Geometry check sheet. Reference: the model listing, model coordinates, mm. Coordinates: 2 decimals unless noted, no trailing zeros. Write each loop counter-clockwise with the first axis right and the second up, starting at its lowest first coordinate (ties: lowest second). Pieces come first, ordered by that corner, then holes. Notation, with made-up numbers: M -0.5,0 L 18.5,0 A38 cw 18.5,38 Z; hole C 13,-30.5 d11. An arc over 180 degrees is marked long. Put each result on its own line as item: value. Start each with the question number.
1) Cross-section at B-B on x = 11. Record the cut outline in (y, z).
2) Cross-section at A-A on y = 2. Record the cut outline in (x, z).
3) Gauge pin test, flat end, axial feed: pin 1 (1.8 mm diameter, centred on x = -7.78, y = 7.78, fed in from +Z). Record the tip position at first contact, or that the pin passes through.
4) Cross-section at C-C on z = 0.4. Count the separate pieces of the cut face and the enclosed holes in it, plus the area to 3 significant figures.
5) Cross-section at D-D on x = 1. Record the cut outline in (y, z), plus the area to 3 significant figures.
6) Scan lines: line 1 along Y through (x, z) = (0, 0.2); line 2 along X through (y, z) = (7.5, 0.2); line 3 along X through (y, z) = (-1, 0.5). Record each from-to range of solid material in increasing order.
Autodesk Inventor part; units mm, degrees
ref_plane "YZ Plane" through (0, 0, 0) normal (1, 0, 0) x (0, 1, 0)
ref_plane "XZ Plane" through (0, 0, 0) normal (0, 1, 0) x (-1, 0, 0)
ref_plane "XY Plane" through (0, 0, 0) normal (0, 0, 1) x (1, 0, 0)
sketch "Sketch1" plane through (0, 0, 0) normal (0, 0, 1) x (1, 0, 0)
  line L0 (-13, -11) -> (13, -11) construction
  circle A0 centre (0, 0) radius 13.8 construction
  circle A1 centre (0, 0) radius 5 construction
  circle A2 centre (0, -11) radius 1.2813 construction
  circle A3 centre (-7.7782, -7.7782) radius 1.2813 construction
  circle A4 centre (-11, 0) radius 1.2813 construction
  circle A5 centre (-7.7782, 7.7782) radius 1.2813 construction
  circle A6 centre (0, 11) radius 1.2813 construction
  circle A7 centre (7.7782, 7.7782) radius 1.2813 construction
  circle A8 centre (11, 0) radius 1.2813 construction
  circle A9 centre (7.7782, -7.7782) radius 1.2813 construction
  circle A10 centre (0, -8) radius 1.2 construction
  circle A11 centre (-8, 0) radius 1.2 construction
  circle A12 centre (0, 8) radius 1.2 construction
  circle A13 centre (8, 0) radius 1.2 construction
  circle A14 centre (0, -11) radius 1.5
  circle A15 centre (7.7782, -7.7782) radius 1.5
  circle A16 centre (11, 0) radius 1.5
  circle A17 centre (7.7782, 7.7782) radius 1.5
  circle A18 centre (0, 11) radius 1.5
  circle A19 centre (-7.7782, 7.7782) radius 1.5
  circle A20 centre (-11, 0) radius 1.5
  circle A21 centre (-7.7782, -7.7782) radius 1.5
  circle A22 centre (0, 0) radius 6
  circle A23 centre (0, 0) radius 19
  dimension "d0" = 3
  dimension "d3" = 360
  dimension "d5" = 12
  dimension "d6" = 38
extrude "Extrusion1" add sketch "Sketch1" along normal blind 1.1
properties part number "motor_spacer_leg"
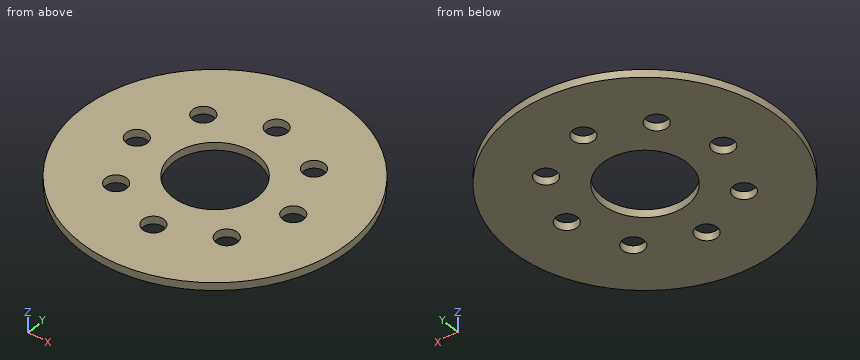
Answer key:
1. outline: M -15.49,0 L -1.5,0 L -1.5,1.1 L -15.49,1.1 Z; M 1.5,0 L 15.49,0 L 15.49,1.1 L 1.5,1.1 Z
2. outline: M -18.89,0 L -5.66,0 L -5.66,1.1 L -18.89,1.1 Z; M 5.66,0 L 18.89,0 L 18.89,1.1 L 5.66,1.1 Z
3. pin 1: passes through
4. separate pieces: 1
4. enclosed holes: 9
4. area: 964 mm²
5. outline: M -18.97,0 L -12.12,0 L -12.12,1.1 L -18.97,1.1 Z; M -9.88,0 L -5.92,0 L -5.92,1.1 L -9.88,1.1 Z; M 5.92,0 L 9.88,0 L 9.88,1.1 L 5.92,1.1 Z; M 12.12,0 L 18.97,0 L 18.97,1.1 L 12.12,1.1 Z
5. area: 23.8 mm²
6. line 1: y = -19 to -12.5, -9.5 to -6, 6 to 9.5, 12.5 to 19
6. line 2: x = -17.46 to -9.25, -6.3 to 6.3, 9.25 to 17.46
6. line 3: x = -18.97 to -12.12, -9.88 to -5.92, 5.92 to 9.88, 12.12 to 18.97
